Verification items for the finished model (mm, model axes). A direction names the side the tool comes from. Give positions to 0.01 mm unless a question says otherwise; leave off trailing zeros. Write each loop counter-clockwise with the first axis right and the second up, starting at its lowest first coordinate (ties: lowest second). Pieces come first, ordered by that corner, then holes. Notation, with made-up numbers: (-31.5, 28.5) -> (13.5, 28.5) arc R17 cw to (13.5, 61.5) -> close; hole circle Ø3 at (-0.5, 22). An arc over 180 degrees is marked (long way). Answer as CSV lines item,"result". Start each with the question number.
1) Material ranges on L1, parallel to Y at x = 2, z = 5.5 (3 decimals); L2, parallel to Z at x = 0, y = -2; L3, parallel to Z at x = 0, y = -51.5, recorded low to high.
2) Sectioned sample at C-C on y = -24.5. Record the cut outline in (x, z) (1 decimal).
3) Mould release check, pull along Z, two halves, no side actions. Record for faces 1 (the cylindrical face through (-13.858, -43.917, 10.626)), 2 (the cylindrical face through (-14.274, -43.418, 0.628)), 3 (the flat face through (5, 0, 0)): released by +Z, released by -Z, zero draft, split by the parting line, or undercut.
4) Gauge pin test, flat ends, axial feed: pin 1 Ø5 at (x, y) = (0.5, -67.5) entering from -Z; pin 2 Ø12 at (x, y) = (9.5, -71.5) entering from +Z; pin 3 Ø3 at (x, z) = (11.5, -10) entering from +Y; pin 4 Ø11 at (x, z) = (0, 0) entering from -Y (3 decimals). Record the tip position at first contact, or that the pin passes through.
5) Tool access check on faces 4 (the flat face through (0, -3.175, -6)), 5 (the cylindrical face through (-3.78, -1.57, 2.9)). Record the directions out of +Z, -Z, +X, -X, +Y, -Y that give a thin tool (end or side, any length) a straight path to the whole face; none if there is none.
```python
from build123d import *

# Parameters (mm, degrees)
SKETCH1_R           = 17.4625
BOSS_EXTRUDE1_DEPTH = 82.55
SKETCH2_R           = 14.2875
CUT_EXTRUDE1_DEPTH  = 79.375
SKETCH3_R           = 4.7625
CUT_EXTRUDE2_DEPTH  = 83.55
FILLET2_R           = 6.35


with BuildPart() as part:
    # Sketch1 → Boss-Extrude1 (new body)
    with BuildSketch(Plane(origin=(0, 0, 0), x_dir=(1, 0, 0), z_dir=(0, 1, 0))):
        Circle(SKETCH1_R)
    extrude(amount=-BOSS_EXTRUDE1_DEPTH)

    # Sketch2 → Cut-Extrude1 (cut)
    with BuildSketch(Plane.XZ.offset(82.55)):
        Circle(SKETCH2_R)
    extrude(amount=-CUT_EXTRUDE1_DEPTH, mode=Mode.SUBTRACT)

    # Sketch3 → Cut-Extrude2 (cut, through all)
    with BuildSketch(Plane(origin=(0, 0, 0), x_dir=(1, 0, 0), z_dir=(0, 1, 0))):
        Circle(SKETCH3_R)
    extrude(amount=-CUT_EXTRUDE2_DEPTH, mode=Mode.SUBTRACT)

    # Fillet2
    fillet2_edges = [part.edges().sort_by_distance(p)[0] for p in [
        (-17.4625, 0, 0),
    ]]
    fillet(fillet2_edges, radius=FILLET2_R)


solid = part.part
```
Ans:
1,L1,"y = -3.175 to 0"
1,L2,"z = -15.74 to -4.76, 4.76 to 15.74"
1,L3,"z = -17.46 to -14.29, 14.29 to 17.46"
2,outline,"circle Ø34.9 at (0, 0); hole circle Ø28.6 at (0, 0)"
3,face 1,"split by the parting line"
3,face 2,"undercut"
3,face 3,"zero draft"
4,pin 1,"stops at z = -17.46"
4,pin 2,"stops at z = 17.11"
4,pin 3,"stops at y = -0.57"
4,pin 4,"stops at y = -3.175"
5,face 4,"-Y"
5,face 5,"+Y, -Y"
